Work out the finished part from the listing and answer in its coordinate system (mm). A direction names the side the tool comes from. Round coordinates to 2 decimals unless told otherwise and drop trailing zeros. Order: outer loops, then holes, each group sorted by start corner. A loop starts at its lowest first (then second) coordinate and runs counter-clockwise, first axis right, second up. Notation, with made-up numbers: (50.25, 8.25) - (72.25, 8.25) arc R17 ccw to (72.25, 41.25) - close; hole circle Ø2 at (77, 11.25). An arc over 180 degrees is marked (long way). Use CSV: the item, a comma, the result in double quotes.
from build123d import *

# Parameters (mm, degrees)
SKETCH4_W           = 32
SKETCH4_H           = 23
BOSS_EXTRUDE3_DEPTH = 19.5
SKETCH5_W           = 29
SKETCH5_H           = 20
CUT_EXTRUDE2_DEPTH  = 8
SKETCH7_W           = 10
SKETCH7_H           = 7
CUT_EXTRUDE4_DEPTH  = 40.198214245
SKETCH8_W           = 32
SKETCH8_H           = 23
BOSS_EXTRUDE4_DEPTH = 10
SKETCH12_R          = 2.6
CUT_EXTRUDE5_DEPTH  = 7
CIRPATTERN1_COUNT   = 2
CIRPATTERN1_ANGLE   = 180
SKETCH13_W          = 15
SKETCH13_H          = 2.791622882
CUT_EXTRUDE6_DEPTH  = 7.1
SKETCH14_W          = 32
SKETCH14_H          = 23
BOSS_EXTRUDE5_DEPTH = 5
BOSS_EXTRUDE6_DEPTH = 32
SKETCH16_R          = 1.7
CUT_EXTRUDE7_DEPTH  = 60.805016512


with BuildPart() as part:
    # Sketch4 → Boss-Extrude3 (new body)
    with BuildSketch(Plane(origin=(0, 0, 0), x_dir=(1, 0, 0), z_dir=(0, 1, 0))):
        Rectangle(SKETCH4_W, SKETCH4_H)
    extrude(amount=BOSS_EXTRUDE3_DEPTH)

    # Sketch5 → Cut-Extrude2 (cut)
    with BuildSketch(Plane(origin=(0, 19.5, 0), x_dir=(1, 0, 0), z_dir=(0, 1, 0))):
        Rectangle(SKETCH5_W, SKETCH5_H)
    extrude(amount=-CUT_EXTRUDE2_DEPTH, mode=Mode.SUBTRACT)

    # Sketch7 → Cut-Extrude4 (cut, through all)
    with BuildSketch(Plane(origin=(16, 0, 0), x_dir=(0, 0, -1), z_dir=(1, 0, 0))):
        with Locations((0, 16)):
            Rectangle(SKETCH7_W, SKETCH7_H)
    extrude(amount=-CUT_EXTRUDE4_DEPTH, mode=Mode.SUBTRACT)

    # Sketch8 → Boss-Extrude4 (add)
    with BuildSketch(Plane(origin=(0, 0, 0), x_dir=(-1, 0, 0), z_dir=(0, -1, 0))):
        Rectangle(SKETCH8_W, SKETCH8_H)
    extrude(amount=BOSS_EXTRUDE4_DEPTH)

    # Sketch12 → Cut-Extrude5 (cut)
    with BuildSketch(Plane(origin=(0, 0, -11.5), x_dir=(-1, 0, 0), z_dir=(0, 0, -1))):
        with Locations((-12.5, -5.726898225)):
            Circle(SKETCH12_R)
        with Locations(Location((-3.5, -5.726898225, 0), (0, 0, 180))):
            Circle(SKETCH12_R)
        with Locations((3.5, -5.726898225)):
            Circle(SKETCH12_R)
        with Locations(Location((12.5, -5.726898225, 0), (0, 0, 180))):
            Circle(SKETCH12_R)
    cut_extrude5 = extrude(amount=-CUT_EXTRUDE5_DEPTH, mode=Mode.SUBTRACT)

    # CirPattern1: Cut-Extrude5 ×2 about axis
    cirpattern1_axis = Axis((0, 11.5, 0), (0, -1, 0))
    for i in range(1, CIRPATTERN1_COUNT):
        add(cut_extrude5.rotate(cirpattern1_axis, i * CIRPATTERN1_ANGLE / (CIRPATTERN1_COUNT - 1)), mode=Mode.SUBTRACT)

    # Sketch13 → Cut-Extrude6 (cut)
    with BuildSketch(Plane(origin=(0, -10, 0), x_dir=(-1, 0, 0), z_dir=(0, -1, 0))):
        with Locations((8.5, 3.895811441)):
            Rectangle(SKETCH13_W, SKETCH13_H)
        with Locations((-8.5, 3.895811441)):
            Rectangle(SKETCH13_W, SKETCH13_H)
        with Locations((-8.5, -3.895811441)):
            Rectangle(SKETCH13_W, SKETCH13_H)
        with Locations((8.5, -3.895811441)):
            Rectangle(SKETCH13_W, SKETCH13_H)
    extrude(amount=-CUT_EXTRUDE6_DEPTH, mode=Mode.SUBTRACT)

    # Sketch14 → Boss-Extrude5 (add)
    with BuildSketch(Plane(origin=(0, -10, 0), x_dir=(-1, 0, 0), z_dir=(0, -1, 0))):
        Rectangle(SKETCH14_W, SKETCH14_H)
    extrude(amount=BOSS_EXTRUDE5_DEPTH)

    # Sketch15 → Boss-Extrude6 (add)
    with BuildSketch(Plane.ZY.offset(16)):
        Polygon((-24.6, -15), (-24.6, -30), (-19.6, -30), (-19.6, -20), (19.6, -20), (19.6, -30), (24.6, -30), (24.6, -15), (11.5, -10), (11.5, -15), (-11.5, -15), (-11.5, -10), align=None)
    extrude(amount=-BOSS_EXTRUDE6_DEPTH)

    # Sketch16 → Cut-Extrude7 (cut, through all)
    with BuildSketch(Plane(origin=(0, 0, -24.6), x_dir=(-1, 0, 0), z_dir=(0, 0, -1))):
        with Locations((7, -25.2)):
            Circle(SKETCH16_R)
        with Locations((-7, -25.2)):
            Circle(SKETCH16_R)
    extrude(amount=-CUT_EXTRUDE7_DEPTH, mode=Mode.SUBTRACT)


solid = part.part
(1) Find section C-C (z = 8.5). Determine the outline of the cut face in (x, y), and give its area (3 significant figures).
Findings below:
outline,"(-16, -20) - (16, -20) - (16, 19.5) - (14.5, 19.5) - (14.5, 11.5) - (-14.5, 11.5) - (-14.5, 19.5) - (-16, 19.5) - close; hole circle Ø5.2 at (-12.5, -5.73); hole circle Ø5.2 at (-3.5, -5.73); hole circle Ø5.2 at (3.5, -5.73); hole circle Ø5.2 at (12.5, -5.73)"
area,"947 mm²"
(2) Find the intervals of material crossed by L1, parallel to Z at x = -6, y = -9; L2, parallel to Z at x = -8, y = 13.5; L3, parallel to Z at x = -12, y = 2, in increasing order. Write a range as from..to.
Findings below:
L1,"z = -11.5..-5.29, -2.5..2.5, 5.29..11.5"
L2,"z = -11.5..-10, 10..11.5"
L3,"z = -11.5..11.5"
(3) Each of these flat-tipped pins is pushed along its axis until it touches: pin 1 (2 mm diameter, centred on x = 2, y = 13.5, fed in from +Z); pin 2 (3 mm diameter, centred on x = 10.5, z = -4.5, fed in from -Y); pin 3 (3 mm diameter, centred on x = 7, y = -25.2, fed in from -Z); pin 4 (0.8 mm diameter, centred on x = -8, z = 3.5, fed in from +Y). Where does it stop, or does it pass through?
Findings below:
pin 1,"stops at z = 11.5"
pin 2,"stops at y = -20"
pin 3,"passes through"
pin 4,"stops at y = 11.5"
(4) Find section D-D (z = -0.5). Determine the outline of the cut face in (x, y).
Findings below:
outline,"(-16, -20) - (16, -20) - (16, 12.5) - (14.5, 12.5) - (14.5, 11.5) - (-14.5, 11.5) - (-14.5, 12.5) - (-16, 12.5) - close"
(5) For faces 4 (the flat face through (-8, -10, -4)), 5 (the cylindrical face through (10.1, -4.73, 8.44)), 6 (the flat face through (9, -2.9, -4)), determine the directions among +Z, -Z, +X, -X, +Y, -Y from which every point of the face is accessible in a straight line to the end or side of a thin tool.
Findings below:
face 4,"-X"
face 5,"+Z"
face 6,"+X"
(6) The mould has two halves that part along X. Classify faces 1 (the flat face through (-1, -6, 4)), 2 (the flat face through (14.5, 12, 0)), 3 (the flat face through (0, -30, -22)): released by +X, released by -X, zero draft, split by the parting line, or undercut.
Findings below:
face 1,"released by -X"
face 2,"undercut"
face 3,"zero draft"
(7) Find section A-A (x = 7). State how many separate pieces and enclosed holes the cut face has, and give its area (3 significant figures).
Findings below:
separate pieces,"3"
enclosed holes,"2"
area,"971 mm²"
